For this review, use the dimensioned drawing (mm, ordinates from the lowest corner) and the shaded views. Round coordinates to 2 decimals unless told otherwise and drop trailing zeros. Write each loop counter-clockwise with the first axis right and the second up, starting at its lowest first coordinate (ties: lowest second). Pieces come first, ordered by that corner, then holes. Notation, with made-up numbers: (69, -3) -> (118, -3) arc R19 cw to (118, 26) -> close; hole circle Ø11 at (-15, 8.5). An arc over 180 degrees is marked (long way). Answer as CSV lines item,"result". Start each with the question number.
Item 1: Wall thickness on probe 1 along Y at (x, z) = (12, 1.4); probe 2 along Y at (x, z) = (11, 3.55); probe 3 along Y at (x, z) = (5, 4.65): over which ranges is each line inside the solid? List them lowest first. Write a range as from..to.
Item 2: Take a section at C-C on z = 3.9. Give the boundary of the cut face in (x, y), then the cut area to 3 significant figures.
Item 3: Take a section at D-D on y = 63. Give the boundary of the cut face in (x, z), then the cut area to 3 significant figures.
Item 4: Take a section at B-B on y = 20. Give the boundary of the cut face in (x, z).
Item 5: Take a section at A-A on x = 12. Give the boundary of the cut face in (y, z).
Item 6: For pin 1 Ø1 at (y, z) = (65.5, 4.5) entering from +X; pin 2 Ø2 at (x, z) = (18, 4) entering from -Y; pin 3 Ø3 at (x, z) = (16.5, 4.5) entering from -Y, all flat-tipped, find the tip position at first contact; note any pin that passes through.
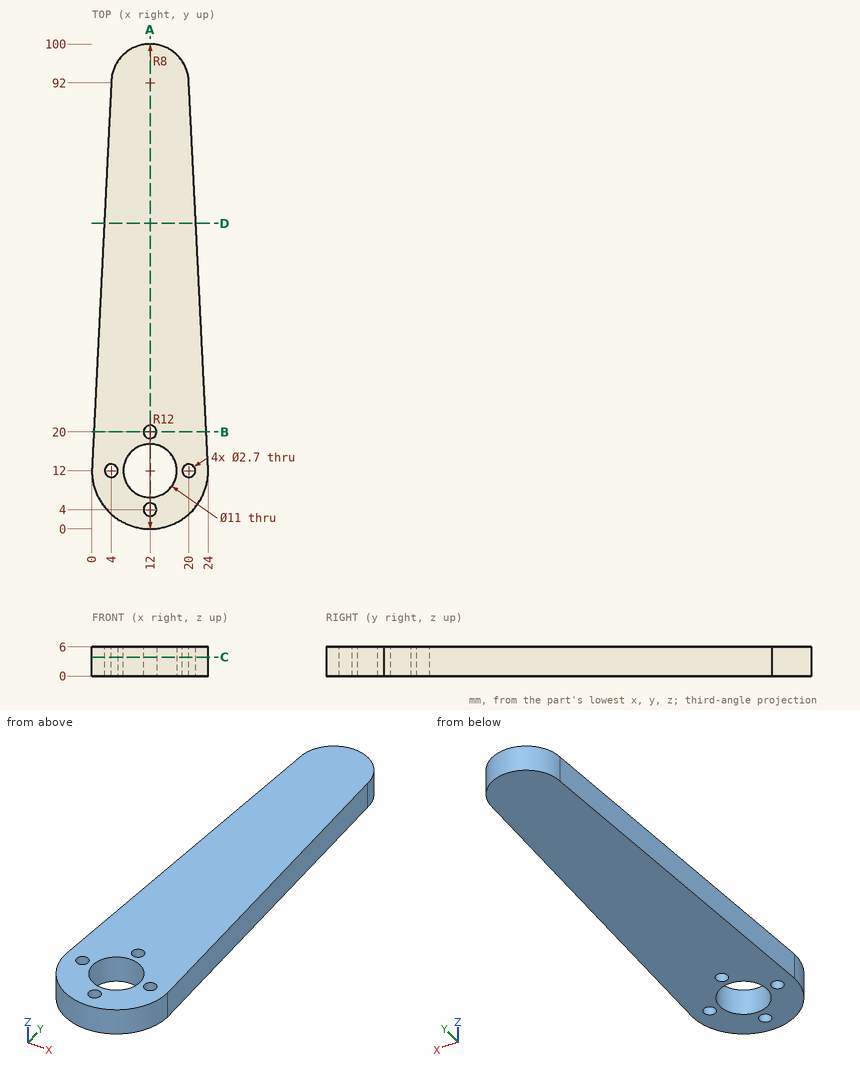
Output values:
1,probe 1,"y = 0..2.65, 5.35..6.5, 17.5..18.65, 21.35..100"
1,probe 2,"y = 0.04..3.09, 4.91..6.59, 17.41..19.09, 20.91..99.94"
1,probe 3,"y = 2.25..11.09, 12.91..95.87"
2,outline,"(0, 12) arc R12 ccw to (24, 12) -> (20, 92) arc R8 ccw to (4, 92) -> close; hole circle Ø2.7 at (4, 12); hole circle Ø11 at (12, 12); hole circle Ø2.7 at (12, 4); hole circle Ø2.7 at (12, 20); hole circle Ø2.7 at (20, 12)"
2,area,"1,810 mm^2"
3,outline,"(2.55, 0) -> (21.45, 0) -> (21.45, 6) -> (2.55, 6) -> close"
3,area,"113 mm^2"
4,outline,"(0.4, 0) -> (10.65, 0) -> (10.65, 6) -> (0.4, 6) -> close; (13.35, 0) -> (23.6, 0) -> (23.6, 6) -> (13.35, 6) -> close"
5,outline,"(0, 0) -> (2.65, 0) -> (2.65, 6) -> (0, 6) -> close; (5.35, 0) -> (6.5, 0) -> (6.5, 6) -> (5.35, 6) -> close; (17.5, 0) -> (18.65, 0) -> (18.65, 6) -> (17.5, 6) -> close; (21.35, 0) -> (100, 0) -> (100, 6) -> (21.35, 6) -> close"
6,pin 1,"stops at x = 21.35"
6,pin 2,"stops at y = 1.09"
6,pin 3,"stops at y = 0.38"
